```python
from build123d import *

# Parameters (mm, degrees)
F0_R     = 12.7
F1_DEPTH = 12.7


# Not quite as in the source:
# - a length typed as a fraction of an inch, garbled in the dataset ("3 / 203.2 mm" for 3/8 in), is restored


with BuildPart() as f1:
    # F0 (on Right) → F1 (new body)
    with BuildSketch(Plane.YZ):
        with BuildLine():
            ThreePointArc((36.9027980984, -24.1696875), (19.129375, 0), (36.9027980984, 24.1696875))
            Line((36.9027980984, 24.1696875), (-67.7783956954, 39.131875))
            ThreePointArc((-67.7783956954, 39.131875), (-78.26375, 0), (-67.7783956954, -39.131875))
            Line((-67.7783956954, -39.131875), (36.9027980984, -24.1696875))
        make_face()
        Circle(F0_R, mode=Mode.SUBTRACT)
        with BuildLine():
            ThreePointArc((36.9027980984, -24.1696875), (59.4505696765, -20.3989450651), (69.770625, 0))
            ThreePointArc((69.770625, 0), (59.4505696765, 20.3989450651), (36.9027980984, 24.1696875))
            ThreePointArc((36.9027980984, 24.1696875), (19.129375, 0), (36.9027980984, -24.1696875))
        make_face()
        with Locations((44.45, 0)):
            Circle(F0_R, mode=Mode.SUBTRACT)
    extrude(amount=F1_DEPTH)


solid = f1.part
```
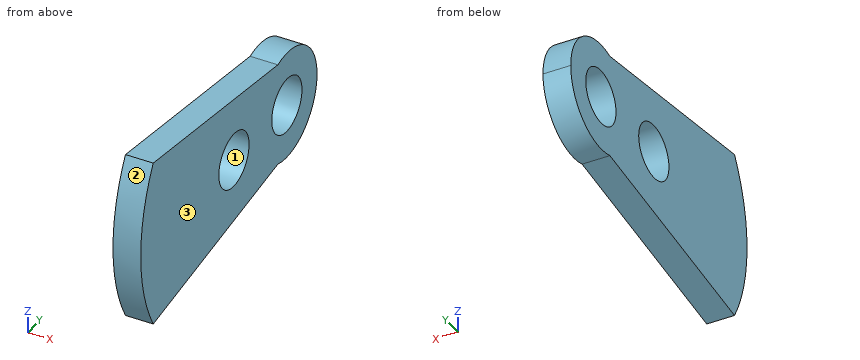
Geometry: final body of the model. Coordinates: model frame, mm. Face numbers are marked on the shaded views. Give positions to 0.01 mm unless a question says otherwise; leave off trailing zeros. Loops run counter-clockwise (first coordinate to the right, second up) from the corner with the lowest first, then second, coordinate; pieces in that order, holes last. Notation, with made-up numbers: (-15.75, -18.5) -> (-7.75, -18.5) arc R32 cw to (-7.75, 12.5) -> close; hole circle Ø8 at (74.25, 63.25). An arc over 180 degrees is marked (long way). Return JSON: item names as keys, results as strings.
Item 1: Section A-A, the plane y = 44.45. Output: boundary loops of the cut face in (x, z), plus the area to 3 significant figures.
Filled in:
{"outline": "(0, -25.32) -> (12.7, -25.32) -> (12.7, -12.7) -> (0, -12.7) -> close; (0, 12.7) -> (12.7, 12.7) -> (12.7, 25.32) -> (0, 25.32) -> close", "area": "321 mm^2"}
Item 2: Line query: line 1 (Z direction, x = 6, y = 44.45); line 2 (Y direction, x = 9.5, z = 8); line 3 (Z direction, x = 6.25, y = 0). Output: solid intervals per line, ascending.
Filled in:
{"line 1": "-25.32 to -12.7, 12.7 to 25.32", "line 2": "-77.85 to -9.86, 9.86 to 34.59, 54.31 to 68.47", "line 3": "-29.44 to -12.7, 12.7 to 29.44"}
Item 3: Section D-D, the plane y = 0. Output: boundary loops of the cut face in (x, z), plus the area to 3 significant figures.
Filled in:
{"outline": "(0, -29.44) -> (12.7, -29.44) -> (12.7, -12.7) -> (0, -12.7) -> close; (0, 12.7) -> (12.7, 12.7) -> (12.7, 29.44) -> (0, 29.44) -> close", "area": "425 mm^2"}
Item 4: Mould query, pull axis Y, two halves, no side actions, for the marked faces 1, 2 and 3. Classes: released by +Y, released by -Y, zero draft, split by the parting line, or undercut.
Filled in:
{"face 1": "undercut", "face 2": "released by -Y", "face 3": "zero draft"}
Item 5: Section C-C, the plane z = 11. Output: boundary loops of the cut face in (x, y), plus the area to 3 significant figures.
Filled in:
{"outline": "(0, -77.49) -> (12.7, -77.49) -> (12.7, -6.35) -> (0, -6.35) -> close; (0, 6.35) -> (12.7, 6.35) -> (12.7, 38.1) -> (0, 38.1) -> close; (0, 50.8) -> (12.7, 50.8) -> (12.7, 67.26) -> (0, 67.26) -> close", "area": "1,520 mm^2"}
Item 6: Pin query (flat end, axial travel): P1, Ø4, axis at x = 4.5, z = 4.5, coming from the +Y side; P2, Ø1.5, axis at x = 5.5, z = -21, coming from the -Y side; P3, Ø15, axis at y = 0, z = 0, coming from the -X side; P4, Ø2, axis at x = 10.5, y = -28.5, coming from the -Z side. Return the tip coordinate at first contact, or that it passes through.
Filled in:
{"P1": "y = 69.65", "P2": "y = -75.6", "P3": "through", "P4": "z = -33.66"}
Item 7: Section B-B, the plane x = 5.5. Output: boundary loops of the cut face in (y, z), plus the area to 3 significant figures.
Filled in:
{"outline": "(-67.78, -39.13) -> (36.9, -24.17) arc R25.32 ccw (long way) to (36.9, 24.17) -> (-67.78, 39.13) arc R78.26 ccw to start; hole circle Ø25.4 at (0, 0); hole circle Ø25.4 at (44.45, 0)", "area": "7,550 mm^2"}
